Design review of the part built by this model. Coordinates are the model's own, in mm. A direction names the side the tool comes from. Give positions to 0.01 mm unless a question says otherwise; leave off trailing zeros. Order: outer loops, then holes, each group sorted by start corner. A loop starts at its lowest first (then second) coordinate and runs counter-clockwise, first axis right, second up. Notation, with made-up numbers: (73, 40.25) -> (122, 40.25) arc R29 ccw to (122, 73.25) -> close; hole circle Ø2 at (57, -14.5). An arc over 180 degrees is marked (long way). Answer in a Markdown table with one row per item. Add a question column.
```python
from build123d import *

# Parameters (mm, degrees)
SKETCH_W        = 54
SKETCH_H        = 68
PAD_DEPTH       = 24
SKETCH001_W     = 51
SKETCH001_H     = 45
POCKET_DEPTH    = 22.5
SKETCH002_W     = 51
SKETCH002_H     = 19.5
POCKET001_DEPTH = 18.5


with BuildPart() as part:
    # Sketch → Pad (new body)
    with BuildSketch(Plane.XY):
        with Locations((27, 34)):
            Rectangle(SKETCH_W, SKETCH_H)
    extrude(amount=PAD_DEPTH)

    # Sketch001 (on Face6 of Pad) → Pocket (cut)
    with BuildSketch(Plane.XY.offset(24)):
        with Locations((27, 44)):
            Rectangle(SKETCH001_W, SKETCH001_H)
    extrude(amount=-POCKET_DEPTH, mode=Mode.SUBTRACT)

    # Sketch002 (on Face5 of Pocket) → Pocket001 (cut)
    with BuildSketch(Plane.XY.offset(24)):
        with Locations((27, 11.25)):
            Rectangle(SKETCH002_W, SKETCH002_H)
    extrude(amount=-POCKET001_DEPTH, mode=Mode.SUBTRACT)


solid = part.part
```
1) For L1, parallel to Y at x = 51.5, z = 13.75; L2, parallel to X at y = 28, z = 19; L3, parallel to Y at x = 20, z = 2.25, list the stretches that pass through material, from the lowest coordinate up.
2) Mouldability with a two-part tool opening along X and no side actions: class faces 1 (the face through (0, 34, 12)), 2 (the face through (1.5, 44, 13)), 3 (the face through (27, 68, 12)), 4 (the face through (27, 21.5, 13)) as +X half, -X half, draft (parallel to the pull), parting line (faces both ways), or undercut.
3) Add section A-A, the plane x = 36. Write out the cut boundary in (y, z), and give its area (3 significant figures).
4) Add section D-D, the plane y = 40.5. Write out the cut boundary in (x, z), and give its area (4 significant figures).
5) Add section B-B, the plane z = 16. Write out the cut boundary in (x, y), and give its area (4 significant figures).
6) Add section C-C, the plane y = 18. Write out the cut boundary in (x, z), and give its area (4 significant figures).
7) Clearance check with flat-ended pins moving along their axes: P1, Ø22.5, axis at x = 28, y = 42.5, coming from the +Z side; P2, Ø1.5, axis at x = 22, y = 9.5, coming from the +Z side. State where each tip first meets the part, or that it passes through.
8) Machinability: for faces 5 (the face through (27, 34, 0)), 6 (the face through (52.5, 44, 13)), which of the approach directions +Z, -Z, +X, -X, +Y, -Y give a long, thin tool a straight path to every point of the face, cutting with its end or side? Answer none if there is none.
Verdict:
| question | item | result |
|---|---|---|
| 1 | L1 | y = 0 to 1.5, 21 to 21.5, 66.5 to 68 |
| 1 | L2 | x = 0 to 1.5, 52.5 to 54 |
| 1 | L3 | y = 0 to 21.5, 66.5 to 68 |
| 2 | face 1 | -X half |
| 2 | face 2 | undercut |
| 2 | face 3 | draft |
| 2 | face 4 | undercut |
| 3 | outline | (0, 0) -> (68, 0) -> (68, 24) -> (66.5, 24) -> (66.5, 1.5) -> (21.5, 1.5) -> (21.5, 24) -> (21, 24) -> (21, 5.5) -> (1.5, 5.5) -> (1.5, 24) -> (0, 24) -> close |
| 3 | area | 259 mm2 |
| 4 | outline | (0, 0) -> (54, 0) -> (54, 24) -> (52.5, 24) -> (52.5, 1.5) -> (1.5, 1.5) -> (1.5, 24) -> (0, 24) -> close |
| 4 | area | 148.5 mm2 |
| 5 | outline | (0, 0) -> (54, 0) -> (54, 68) -> (0, 68) -> close; hole (1.5, 1.5) -> (52.5, 1.5) -> (52.5, 21) -> (1.5, 21) -> close; hole (1.5, 21.5) -> (52.5, 21.5) -> (52.5, 66.5) -> (1.5, 66.5) -> close |
| 5 | area | 382.5 mm2 |
| 6 | outline | (0, 0) -> (54, 0) -> (54, 24) -> (52.5, 24) -> (52.5, 5.5) -> (1.5, 5.5) -> (1.5, 24) -> (0, 24) -> close |
| 6 | area | 352.5 mm2 |
| 7 | P1 | stops at z = 1.5 |
| 7 | P2 | stops at z = 5.5 |
| 8 | face 5 | -Z, +X, -X, +Y, -Y |
| 8 | face 6 | +Z |
